Autodesk Inventor part; units mm, degrees
ref_plane "Work Plane1" through (6.223, -18.1368, 0) normal (-1, 0, 0) x (0, 0, 1)
ref_plane "YZ Plane" through (0, 0, 0) normal (1, 0, 0) x (0, 1, 0)
ref_plane "XZ Plane" through (0, 0, 0) normal (0, 1, 0) x (-1, 0, 0)
sketch "Sketch1" plane through (0, 0, 0) normal (0, 0, 1) x (1, 0, 0)
  line L0 (11.176, -4.445) -> (1.27, -4.445)
  line L1 (-5.4348, 0) -> (-5.4348, -19.4068)
  line L2 (12.446, 0) -> (12.446, -11.684)
  line L3 (19.05, -11.684) -> (19.05, -16.51)
  line L4 (19.05, -16.51) -> (12.446, -16.51)
  line L5 (-4.1648, -1.27) -> (0, -1.27)
  line L6 (-4.1648, -18.1368) -> (-4.1648, -1.27)
  line L7 (0, -4.445) -> (0, -1.27)
  line L8 (1.27, -5.715) -> (11.176, -5.715)
  line L9 (11.176, -22.86) -> (1.27, -22.86)
  line L10 (1.27, -18.1368) -> (11.176, -18.1368)
  line L11 (12.446, -15.24) -> (17.78, -15.24)
  line L12 (17.78, -15.24) -> (17.78, -12.954)
  line L13 (17.78, -12.954) -> (12.446, -12.954)
  line L14 (11.176, -5.715) -> (11.176, -18.1368)
  line L15 (12.446, -15.24) -> (12.446, -12.954)
  line L16 (12.446, -15.24) -> (13.462, -15.24) construction
  line L17 (11.176, -4.445) -> (11.176, -1.27)
  line L18 (1.27, -4.445) -> (1.27, -1.27)
  line L19 (0, -18.1368) -> (0, -1.27)
  line L20 (1.27, -1.27) -> (11.176, -1.27)
  line L21 (1.27, -18.1368) -> (1.27, -5.715)
  line L22 (11.176, -22.86) -> (11.176, -19.4068)
  line L23 (1.27, -22.86) -> (1.27, -19.4068)
  line L24 (1.27, -22.86) -> (3.1836, -22.86) construction
  line L25 (12.446, 0) -> (-5.4348, 0)
  line L26 (12.446, -16.51) -> (12.446, -24.13)
  line L27 (0, -18.1368) -> (-4.1648, -18.1368)
  line L28 (12.446, -11.684) -> (19.05, -11.684)
  line L29 (12.446, -24.13) -> (0, -24.13)
  line L30 (0, -24.13) -> (0, -19.4068)
  line L31 (0, -19.4068) -> (-5.4348, -19.4068)
  line L32 (1.27, -19.4068) -> (11.176, -19.4068)
  point P0 (0, 0)
  point P1 (0, -10.414)
  point P2 (-4.1648, -10.414)
extrude "Extrusion1" add sketch "Sketch1" along normal blind 3.8354
sketch "Sketch3" plane through (0, 0, 3.8354) normal (0, 0, 1) x (1, 0, 0)
  line L0 (19.05, -16.51) -> (19.05, -11.684)
  line L1 (19.05, -11.684) -> (12.446, -11.684)
  line L2 (12.446, -11.684) -> (12.446, 0)
  line L3 (12.446, 0) -> (-5.4348, 0)
  line L4 (-5.4348, 0) -> (-5.4348, -19.4068)
  line L5 (-5.4348, -19.4068) -> (0, -19.4068)
  line L6 (0, -19.4068) -> (0, -24.13)
  line L7 (0, -24.13) -> (12.446, -24.13)
  line L8 (12.446, -24.13) -> (12.446, -16.51)
  line L9 (12.446, -16.51) -> (19.05, -16.51)
extrude "Extrusion3" add sketch "Sketch3" along normal blind 1.016
ref_plane "Work Plane1" through (6.223, -18.1368, 0) normal (-1, 0, 0) x (0, 0, 1)
properties part number "Remote Batery Spacer"
Part model, mm, in its own coordinate system. A direction names the side the tool comes from. Round coordinates to 2 decimals unless told otherwise and drop trailing zeros. Write each loop counter-clockwise with the first axis right and the second up, starting at its lowest first coordinate (ties: lowest second). Pieces come first, ordered by that corner, then holes. Notation, with made-up numbers: M -11.5,23 L 11.5,23 A21 cw 11.5,61 Z; hole C 27,24 d4. An arc over 180 degrees is marked long. Answer as CSV lines item,"result". Start each with the question number.
1) Drill centre lines: L1, parallel to X at y = -4, z = 1.25; L2, parallel to X at y = -16, z = 3.1; L3, parallel to Y at x = 10.5, z = 2 (3 decimals). Where is each one in solid material? Low to high.
2) Which spindle directions (+Z, -Z, +X, -X, +Y, -Y) get a long thin tool onto all of the face, cutting with end or side? Do faces 4 (the face through (12.446, -6, 2)), 5 (the face through (0, -22, 2)), 6 (the face through (16, -16.51, 2)), 7 (the face through (6, -18.137, 2)). Say none if no direction does.
3) Band-saw the part on B-B (z = 2.6). Count the separate pieces of the cut face and the enclosed holes in it, then the cut area to 3 significant figures.
4) Band-saw the part on C-C (x = 4.75). List the corners of the cut face in (y, z) (3 decimals), then the cut area to 3 significant figures.
5) Mould opens along Y. For faces 1 (the face through (4, -12, 4.851)), 2 (the face through (11.176, -21, 2)), 3 (the face through (-3, -19.407, 2)) say: +Y half, -Y half, draft (parallel to the pull), parting line (faces both ways), or undercut.
6) Band-saw the part on A-A (y = -10.5). List the corners of the cut face in (x, z), then the cut area to 3 significant figures.
7) Drop flat-ended pins along their axis: pin 1 (2 mm diameter, centred on x = -1.5, y = -7, fed in from -Z); pin 2 (1.6 mm diameter, centred on y = -3, z = 1, fed in from +X); pin 3 (1 mm diameter, centred on x = 14, z = 4.5, fed in from -Y). Give the stop position or say it passes through.
8) Band-saw the part on D-D (z = 4.55). List the corners of the cut face in (x, y).
Worked out:
1,L1,"-5.43 to -4.16, 0 to 1.27, 11.18 to 12.45"
1,L2,"-5.43 to -4.16, 0 to 1.27, 11.18 to 19.05"
1,L3,"-24.13 to -22.86, -19.407 to -18.137, -5.715 to -4.445, -1.27 to 0"
2,face 4,"+Z, -Z, +X, +Y"
2,face 5,"+Z, -Z, -X, -Y"
2,face 6,"+Z, -Z, +X, -Y"
2,face 7,"-Z"
3,separate pieces,"1"
3,enclosed holes,"5"
3,area,"167 mm²"
4,outline,"M -24.13,0 L -22.86,0 L -22.86,3.835 L -19.407,3.835 L -19.407,0 L -18.137,0 L -18.137,3.835 L -5.715,3.835 L -5.715,0 L -4.445,0 L -4.445,3.835 L -1.27,3.835 L -1.27,0 L 0,0 L 0,4.851 L -24.13,4.851 Z"
4,area,"44.0 mm²"
5,face 1,"draft"
5,face 2,"undercut"
5,face 3,"-Y half"
6,outline,"M -5.43,0 L -4.16,0 L -4.16,3.84 L 0,3.84 L 0,0 L 1.27,0 L 1.27,3.84 L 11.18,3.84 L 11.18,0 L 12.45,0 L 12.45,4.85 L -5.43,4.85 Z"
6,area,"32.8 mm²"
7,pin 1,"z = 3.84"
7,pin 2,"x = 12.45"
7,pin 3,"y = -16.51"
8,outline,"M -5.43,-19.41 L 0,-19.41 L 0,-24.13 L 12.45,-24.13 L 12.45,-16.51 L 19.05,-16.51 L 19.05,-11.68 L 12.45,-11.68 L 12.45,0 L -5.43,0 Z"
